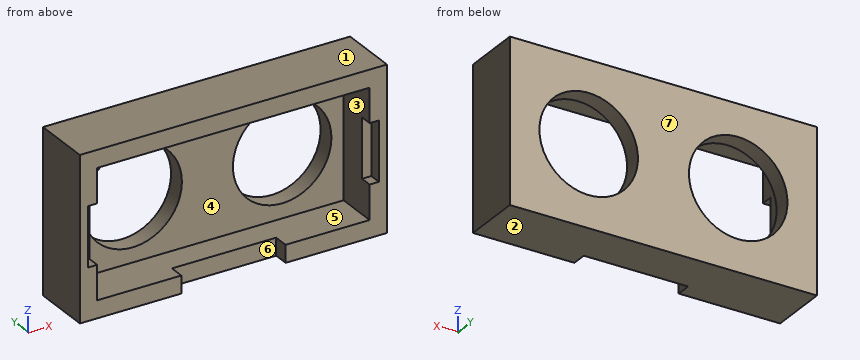
from build123d import *

# Parameters (mm, degrees)
SKETCH2_R           = 3.175
BOSS_EXTRUDE1_DEPTH = 3
SKETCH4_W           = 53
SKETCH4_H           = 25
BOSS_EXTRUDE3_DEPTH = 3
BOSS_EXTRUDE4_DEPTH = 7.2
SKETCH6_R           = 8.5
CUT_EXTRUDE1_DEPTH  = 7.2
SKETCH7_W           = 18
SKETCH7_H           = 6
CUT_EXTRUDE2_DEPTH  = 2.6
SKETCH8_W           = 1.6
SKETCH8_H           = 10.2
CUT_EXTRUDE3_DEPTH  = 2.1
CUT_EXTRUDE4_START  = -3
CUT_EXTRUDE4_DEPTH  = 3


with BuildPart() as part:
    # Sketch2 → Boss-Extrude1 (new body)
    with BuildSketch(Plane.XY):
        with BuildLine():
            Line((26.5, 7.809866434), (26.5, 7.967433715))
            Line((26.5, 7.967433715), (51.343101615, 22.31060512))
            ThreePointArc((51.343101615, 22.31060512), (51.20337497, 29.562282322), (44.993101615, 33.309127748))
            Line((44.993101615, 33.309127748), (18.494003701, 18.009866434))
            Line((18.494003701, 18.009866434), (-18.494003701, 18.009866434))
            Line((-18.494003701, 18.009866434), (-44.993101615, 33.309127748))
            ThreePointArc((-44.993101615, 33.309127748), (-51.20337497, 29.562282322), (-51.343101615, 22.31060512))
            Line((-51.343101615, 22.31060512), (-26.5, 7.967433715))
            Line((-26.5, 7.967433715), (-26.5, 7.809866434))
            Line((-26.5, 7.809866434), (26.5, 7.809866434))
        make_face()
        with Locations((44.704, 25.809866434)):
            Circle(SKETCH2_R, mode=Mode.SUBTRACT)
        with Locations((-44.704, 25.809866434)):
            Circle(SKETCH2_R, mode=Mode.SUBTRACT)
    extrude(amount=BOSS_EXTRUDE1_DEPTH)

    # Sketch4 → Boss-Extrude3 (add)
    with BuildSketch(Plane(origin=(0, 18.009866434, 0), x_dir=(1, 0, 0), z_dir=(0, 1, 0))):
        with Locations((0, -15.5)):
            Rectangle(SKETCH4_W, SKETCH4_H)
    extrude(amount=-BOSS_EXTRUDE3_DEPTH)

    # Sketch5 → Boss-Extrude4 (add)
    with BuildSketch(Plane.XZ.offset(-15.009866434)):
        Polygon((-26.5, 3), (-23.5, 3), (-23.5, 25), (23.5, 25), (23.5, 3), (26.5, 3), (26.5, 28), (-26.5, 28), align=None)
    extrude(amount=BOSS_EXTRUDE4_DEPTH)

    # Sketch6 → Cut-Extrude1 (cut)
    with BuildSketch(Plane.XZ.offset(-15.009866434)):
        with Locations((12.9, 14)):
            Circle(SKETCH6_R)
        with Locations((-12.9, 14)):
            Circle(SKETCH6_R)
    extrude(amount=-CUT_EXTRUDE1_DEPTH, mode=Mode.SUBTRACT)

    # Sketch7 → Cut-Extrude2 (cut)
    with BuildSketch(Plane.XZ.offset(-7.809866434)):
        with Locations((0, 3)):
            Rectangle(SKETCH7_W, SKETCH7_H)
    extrude(amount=-CUT_EXTRUDE2_DEPTH, mode=Mode.SUBTRACT)

    # Sketch8 → Cut-Extrude3 (cut)
    with BuildSketch(Plane.XZ.offset(-7.809866434)):
        with Locations((-24.3, 14)):
            Rectangle(SKETCH8_W, SKETCH8_H)
        with Locations((24.3, 14)):
            Rectangle(SKETCH8_W, SKETCH8_H)
    extrude(amount=-CUT_EXTRUDE3_DEPTH, mode=Mode.SUBTRACT)

    # Sketch11 → Cut-Extrude4 (cut)
    with BuildSketch(Plane.XY.offset(3).offset(CUT_EXTRUDE4_START)):
        with BuildLine():
            Line((-51.343101615, 22.31060512), (-26.5, 7.967433715))
            Line((-26.5, 7.967433715), (-26.5, 18.009866434))
            Line((-26.5, 18.009866434), (-18.494003701, 18.009866434))
            Line((-18.494003701, 18.009866434), (-44.993101615, 33.309127748))
            ThreePointArc((-44.993101615, 33.309127748), (-51.20337497, 29.562282322), (-51.343101615, 22.31060512))
        make_face()
        with BuildLine():
            Line((26.5, 18.009866434), (26.5, 7.967433715))
            Line((26.5, 7.967433715), (51.343101615, 22.31060512))
            ThreePointArc((51.343101615, 22.31060512), (51.20337497, 29.562282322), (44.993101615, 33.309127748))
            Line((44.993101615, 33.309127748), (18.494003701, 18.009866434))
            Line((18.494003701, 18.009866434), (26.5, 18.009866434))
        make_face()
    extrude(amount=CUT_EXTRUDE4_DEPTH, mode=Mode.SUBTRACT)


solid = part.part
Verification items for the finished model (mm, model axes). Face numbers are marked on the shaded views. A direction names the side the tool comes from. Give positions to 0.01 mm unless a question says otherwise; leave off trailing zeros. Loops run counter-clockwise (first coordinate to the right, second up) from the corner with the lowest first, then second, coordinate; pieces in that order, holes last.
1. Go/stop test with a flat-tipped pin: P1, Ø4, axis at x = -1.5, z = 3, coming from the -Y side. Record where the tip stops, or that it passes through.
Derived:
P1: stops at y = 10.41
2. Cross-section at D-D on y = 17. Record the cut outline in (x, z).
Derived:
outline: (-26.5, 0) - (26.5, 0) - (26.5, 28) - (-26.5, 28) - close; hole circle Ø17 at (-12.9, 14); hole circle Ø17 at (12.9, 14)
3. Cross-section at A-A on x = -12.9. Record the cut outline in (y, z).
Derived:
outline: (7.81, 0) - (18.01, 0) - (18.01, 5.5) - (15.01, 5.5) - (15.01, 3) - (7.81, 3) - close; (7.81, 25) - (15.01, 25) - (15.01, 22.5) - (18.01, 22.5) - (18.01, 28) - (7.81, 28) - close
4. Cross-section at B-B on z = 14. Record the cut outline in (x, y), and give its area (3 significant figures).
Derived:
outline: (-26.5, 7.81) - (-25.1, 7.81) - (-25.1, 9.91) - (-23.5, 9.91) - (-23.5, 15.01) - (-21.4, 15.01) - (-21.4, 18.01) - (-26.5, 18.01) - close; (-4.4, 15.01) - (4.4, 15.01) - (4.4, 18.01) - (-4.4, 18.01) - close; (21.4, 15.01) - (23.5, 15.01) - (23.5, 9.91) - (25.1, 9.91) - (25.1, 7.81) - (26.5, 7.81) - (26.5, 18.01) - (21.4, 18.01) - close
area: 93.5 mm2
5. Cross-section at C-C on y = 14.5. Record the cut outline in (x, z), and give its area (3 significant figures).
Derived:
outline: (-26.5, 0) - (26.5, 0) - (26.5, 28) - (-26.5, 28) - close; hole (-23.5, 3) - (23.5, 3) - (23.5, 25) - (-23.5, 25) - close
area: 450 mm2
6. Release check for a two-part mould opening along Z. For the marked faces 1, 2, 3 and 4 record: +Z half, -Z half, draft (parallel to the pull), parting line (faces both ways), or undercut.
Derived:
face 1: +Z half
face 2: -Z half
face 3: undercut
face 4: undercut
7. Material ranges on probe 1 along X at (y, z) = (9.5, 14.5); probe 2 along Z at (x, y) = (-12.9, 16.55); probe 3 along X at (y, z) = (16.25, 10.25), recorded low to high.
Derived:
probe 1: x = -26.5 to -25.1, 25.1 to 26.5
probe 2: z = 0 to 5.5, 22.5 to 28
probe 3: x = -26.5 to -20.53, -5.27 to 5.27, 20.53 to 26.5
8. Tool access check on the marked faces 5, 6 and 7. Record the directions out of +Z, -Z, +X, -X, +Y, -Y that give a thin tool (end or side, any length) a straight path to the whole face; none if there is none.
Derived:
face 5: -Y
face 6: -Z, -Y
face 7: +Z, -Z, +X, -X, +Y
